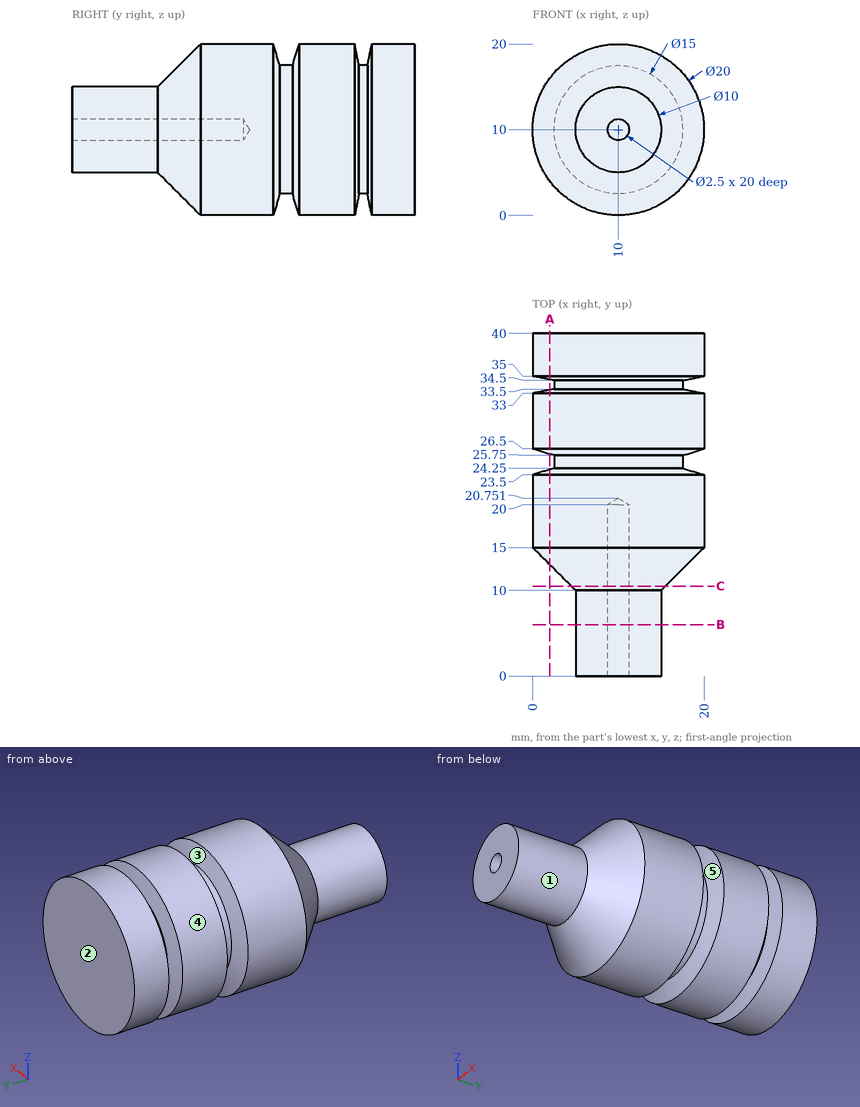
Could you check a few things on this drawing? It's one solid part, dimensions in mm from its lowest x, y, z. A direction names the side the tool comes from. Coordinates: 2 decimals unless noted, no trailing zeros. Order: outer loops, then holes, each group sorted by start corner. A loop starts at its lowest first (then second) coordinate and runs counter-clockwise, first axis right, second up.
1) Imagine slicing it at C-C on y = 10.5. List the corners of the cut face in (x, z) for me, and give its area (3 significant figures).
2) Which directions (+Z, -Z, +X, -X, +Y, -Y) give clear straight access to the entire face, cutting with the end or side of a thin tool? Please do the marked faces 4 and 5.
3) Imagine slicing it at A-A on x = 2. State how many separate pieces and enclosed holes the cut face has, and give its area (3 significant figures).
4) Will these pins go through, and if not, where does the flat tip stop? pin 1 (1.5 mm diameter, centred on x = 3, z = 15, fed in from -Y); pin 2 (2 mm diameter, centred on y = 7, z = 7.5, fed in from -X); pin 3 (1.5 mm diameter, centred on x = 14, y = 20.5, fed in from -Z).
5) I need wall thicknesses on line 1 (Z direction, x = 10, y = 6.75); line 2 (Y direction, x = 8, z = 1.25) (1 decimal). Which ranges of each line are inside material? Lowest first, please.
6) We'd pull the mould along Y, two halves only. Please class the marked faces 1, 2 and 3: +Y half, -Y half, draft (parallel to the pull), parting line (faces both ways), or undercut.
7) Imagine slicing it at B-B on y = 6. List the corners of the cut face in (x, z) for me, and give its area (3 significant figures).
Response values:
1. outline: circle Ø11 at (10, 10); hole circle Ø2.5 at (10, 10)
1. area: 90.1 mm2
2. face 4: +Y, -Y
2. face 5: none
3. separate pieces: 3
3. enclosed holes: 0
3. area: 271 mm2
4. pin 1: stops at y = 12.85
4. pin 2: stops at x = 5.23
4. pin 3: stops at z = 0.54
5. line 1: z = 5 to 8.75, 11.25 to 15
5. line 2: y = 14 to 23.8, 26.2 to 33.2, 34.8 to 40
6. face 1: draft
6. face 2: +Y half
6. face 3: undercut
7. outline: circle Ø10 at (10, 10); hole circle Ø2.5 at (10, 10)
7. area: 73.6 mm2
